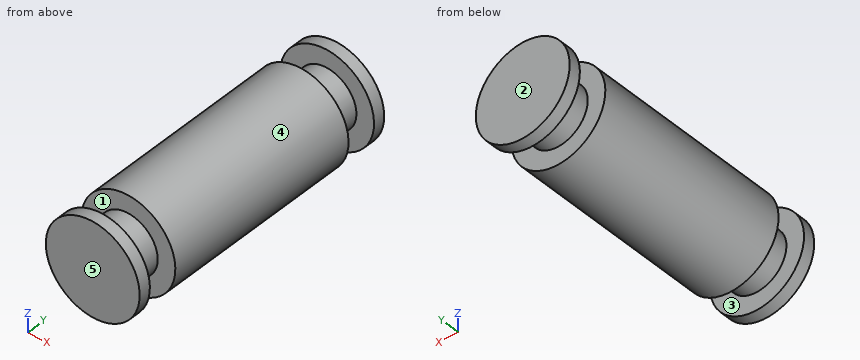
from build123d import *

# Parameters (mm, degrees)
SKETCH1_R           = 4
BOSS_EXTRUDE1_DEPTH = 17
SKETCH2_R           = 2.5
BOSS_EXTRUDE2_DEPTH = 2.5
BOSS_EXTRUDE3_START = 1
SKETCH3_R           = 4
BOSS_EXTRUDE3_DEPTH = 1
BOSS_EXTRUDE4_START = 2.5
SKETCH4_R           = 2.5
BOSS_EXTRUDE4_DEPTH = 2.5
SKETCH5_R           = 4
BOSS_EXTRUDE5_DEPTH = 1


with BuildPart() as part:
    # Sketch1 → Boss-Extrude1 (new body)
    with BuildSketch(Plane(origin=(0, 0, 0), x_dir=(1, 0, 0), z_dir=(0, 1, 0))):
        with Locations(Location((0, 0, 0), (0, 0, 270))):
            Circle(SKETCH1_R)
    extrude(amount=BOSS_EXTRUDE1_DEPTH)

    # Sketch2 → Boss-Extrude2 (add)
    with BuildSketch(Plane.XZ):
        with Locations(Location((0, 0, 0), (0, 0, 270))):
            Circle(SKETCH2_R)
    extrude(amount=BOSS_EXTRUDE2_DEPTH)

    # Sketch3 → Boss-Extrude3 (add)
    with BuildSketch(Plane.XZ.offset(2.5).offset(BOSS_EXTRUDE3_START)):
        with Locations(Location((0, 0, 0), (0, 0, 90))):
            Circle(SKETCH3_R)
    extrude(amount=-BOSS_EXTRUDE3_DEPTH)

    # Sketch4 → Boss-Extrude4 (add)
    with BuildSketch(Plane(origin=(0, 17, 0), x_dir=(1, 0, 0), z_dir=(0, 1, 0)).offset(BOSS_EXTRUDE4_START)):
        with Locations(Location((0, 0, 0), (0, 0, 90))):
            Circle(SKETCH4_R)
    extrude(amount=-BOSS_EXTRUDE4_DEPTH)

    # Sketch5 → Boss-Extrude5 (add)
    with BuildSketch(Plane(origin=(0, 19.5, 0), x_dir=(1, 0, 0), z_dir=(0, 1, 0))):
        with Locations(Location((0, 0, 0), (0, 0, 270))):
            Circle(SKETCH5_R)
    extrude(amount=BOSS_EXTRUDE5_DEPTH)


solid = part.part
Geometry: final body of the model. Coordinates: model frame, mm. Face numbers are marked on the shaded views. A direction names the side the tool comes from. Round coordinates to 2 decimals unless told otherwise and drop trailing zeros. Loops run counter-clockwise (first coordinate to the right, second up) from the corner with the lowest first, then second, coordinate; pieces in that order, holes last. Notation, with made-up numbers: M -20.75,-27 L 27.25,-27 A9 cw 27.25,-13 Z; hole C 46.5,82.5 d3. An arc over 180 degrees is marked long. Put each result on its own line as item: value. Start each with the question number.
(1) Section query A-A (z = 0). Return loops of the section in (x, y), then the cut area to 3 significant figures.
(2) Set-up query: the marked faces 1 and 2. Return all of +Z, -Z, +X, -X, +Y, -Y with unobstructed straight access to the full face (end or side cutting, diameter ignored); none if empty.
(3) Draft query along Y for the marked faces 3, 4 and 5. Return one class per face: +Y half, -Y half, draft (parallel to the pull), parting line (faces both ways), or undercut.
(4) Section query C-C (x = -1.5). Return loops of the section in (y, z).
(5) Section query D-D (y = 2). Return loops of the section in (x, z).
(6) Material intervals for line 1 along Y through (x, z) = (-2.75, 0.75); line 2 along X through (y, z) = (4.25, 3); line 3 along X through (y, z) = (6.25, 1), sorted ascending. Write a range as [from, to].
(7) Contact query for a flat-ended pin moving along its axis: pin 1 Ø1 at (x, y) = (2.5, 8.5) entering from -Z. Output: stop coordinate, or through.
(8) Section query B-B (z = 3). Return loops of the section in (x, y).
Findings below:
1. outline: M -4,-3.5 L 4,-3.5 L 4,-2.5 L 2.5,-2.5 L 2.5,0 L 4,0 L 4,17 L 2.5,17 L 2.5,19.5 L 4,19.5 L 4,20.5 L -4,20.5 L -4,19.5 L -2.5,19.5 L -2.5,17 L -4,17 L -4,0 L -2.5,0 L -2.5,-2.5 L -4,-2.5 Z
1. area: 177 mm2
2. face 1: none
2. face 2: +Z, -Z, +X, -X, +Y
3. face 3: undercut
3. face 4: draft
3. face 5: -Y half
4. outline: M -3.5,-3.71 L -2.5,-3.71 L -2.5,-2 L 0,-2 L 0,-3.71 L 17,-3.71 L 17,-2 L 19.5,-2 L 19.5,-3.71 L 20.5,-3.71 L 20.5,3.71 L 19.5,3.71 L 19.5,2 L 17,2 L 17,3.71 L 0,3.71 L 0,2 L -2.5,2 L -2.5,3.71 L -3.5,3.71 Z
5. outline: C 0,0 d8
6. line 1: y = [-3.5, -2.5], [0, 17], [19.5, 20.5]
6. line 2: x = [-2.65, 2.65]
6. line 3: x = [-3.87, 3.87]
7. pin 1: stops at z = -3.46
8. outline: M -2.65,-3.5 L 2.65,-3.5 L 2.65,-2.5 L -2.65,-2.5 Z; M -2.65,0 L 2.65,0 L 2.65,17 L -2.65,17 Z; M -2.65,19.5 L 2.65,19.5 L 2.65,20.5 L -2.65,20.5 Z
